from build123d import *

# Parameters (mm, degrees)
F0_R     = 45
F1_DEPTH = 8
F3_DEPTH = 25
F5_DEPTH = 25


with BuildPart() as f1:
    # F0 (on Top) → F1 (new body)
    with BuildSketch(Plane.XY):
        Circle(F0_R)
    extrude(amount=F1_DEPTH)

    # F2 (on face) → F3 (cut)
    with BuildSketch(Plane.XY.offset(8)):
        with BuildLine():
            ThreePointArc((-44.7762963998, 4.4814373498), (-31.5268148945, 32.1101221207), (-3.659898693, 44.8509213011))
            Line((-3.659898693, 44.8509213011), (-3.659898693, 46.727180481))
            Line((-3.659898693, 46.727180481), (-14.4028495997, 46.727180481))
            Line((-14.4028495997, 46.727180481), (-30.4222777486, 39.8657522048))
            Line((-30.4222777486, 39.8657522048), (-45.7375533879, 26.1307712644))
            Line((-45.7375533879, 26.1307712644), (-50.4905698847, 4.4814373498))
            Line((-50.4905698847, 4.4814373498), (-44.7762963998, 4.4814373498))
        make_face()
        with BuildLine():
            Line((-3.659898693, 39.8657522048), (-3.659898693, 44.8509213011))
            ThreePointArc((-3.659898693, 44.8509213011), (-31.5268148945, 32.1101221207), (-44.7762963998, 4.4814373498))
            Line((-44.7762963998, 4.4814373498), (-39.7817769409, 4.4814373498))
            Line((-39.7817769409, 4.4814373498), (-38.9415013432, 9.2861472328))
            Line((-38.9415013432, 9.2861472328), (-35.9457781326, 17.6231124305))
            Line((-35.9457781326, 17.6231124305), (-31.6359626456, 24.5324056053))
            Line((-31.6359626456, 24.5324056053), (-25.7671181964, 30.6386794289))
            Line((-25.7671181964, 30.6386794289), (-18.6895557962, 35.4030162759))
            Line((-18.6895557962, 35.4030162759), (-10.3150569916, 38.6816837348))
            Line((-10.3150569916, 38.6816837348), (-3.659898693, 39.8657522048))
        make_face()
        with BuildLine():
            ThreePointArc((44.7762963998, 4.4814373498), (31.5268148945, 32.1101221207), (3.659898693, 44.8509213011))
            Line((3.659898693, 44.8509213011), (3.659898693, 39.8657522048))
            Line((3.659898693, 39.8657522048), (10.3150569916, 38.6816837348))
            Line((10.3150569916, 38.6816837348), (18.6895557962, 35.4030162759))
            Line((18.6895557962, 35.4030162759), (25.7671181964, 30.6386794289))
            Line((25.7671181964, 30.6386794289), (31.6359626456, 24.5324056053))
            Line((31.6359626456, 24.5324056053), (35.9457781326, 17.6231124305))
            Line((35.9457781326, 17.6231124305), (38.9415013432, 9.2861472328))
            Line((38.9415013432, 9.2861472328), (39.7817769409, 4.4814373498))
            Line((39.7817769409, 4.4814373498), (44.7762963998, 4.4814373498))
        make_face()
        with BuildLine():
            Line((3.659898693, 46.727180481), (3.659898693, 44.8509213011))
            ThreePointArc((3.659898693, 44.8509213011), (31.5268148945, 32.1101221207), (44.7762963998, 4.4814373498))
            Line((44.7762963998, 4.4814373498), (50.4905698847, 4.4814373498))
            Line((50.4905698847, 4.4814373498), (45.7375533879, 26.1307712644))
            Line((45.7375533879, 26.1307712644), (30.4222777486, 39.8657522048))
            Line((30.4222777486, 39.8657522048), (14.4028495997, 46.727180481))
            Line((14.4028495997, 46.727180481), (3.659898693, 46.727180481))
        make_face()
        with BuildLine():
            ThreePointArc((3.659898693, -44.8509213011), (31.5268148945, -32.1101221207), (44.7762963998, -4.4814373498))
            Line((44.7762963998, -4.4814373498), (39.7817769409, -4.4814373498))
            Line((39.7817769409, -4.4814373498), (38.9415013432, -9.2861472328))
            Line((38.9415013432, -9.2861472328), (35.9457781326, -17.6231124305))
            Line((35.9457781326, -17.6231124305), (31.6359626456, -24.5324056053))
            Line((31.6359626456, -24.5324056053), (25.7671181964, -30.6386794289))
            Line((25.7671181964, -30.6386794289), (18.6895557962, -35.4030162759))
            Line((18.6895557962, -35.4030162759), (10.3150569916, -38.6816837348))
            Line((10.3150569916, -38.6816837348), (3.659898693, -39.8657522048))
            Line((3.659898693, -39.8657522048), (3.659898693, -44.8509213011))
        make_face()
        with BuildLine():
            Line((50.4905698847, -4.4814373498), (44.7762963998, -4.4814373498))
            ThreePointArc((44.7762963998, -4.4814373498), (31.5268148945, -32.1101221207), (3.659898693, -44.8509213011))
            Line((3.659898693, -44.8509213011), (3.659898693, -46.727180481))
            Line((3.659898693, -46.727180481), (14.4028495997, -46.727180481))
            Line((14.4028495997, -46.727180481), (30.4222777486, -39.8657522048))
            Line((30.4222777486, -39.8657522048), (45.7375533879, -26.1307712644))
            Line((45.7375533879, -26.1307712644), (50.4905698847, -4.4814373498))
        make_face()
        with BuildLine():
            Line((-39.7817769409, -4.4814373498), (-44.7762963998, -4.4814373498))
            ThreePointArc((-44.7762963998, -4.4814373498), (-31.5268148945, -32.1101221207), (-3.659898693, -44.8509213011))
            Line((-3.659898693, -44.8509213011), (-3.659898693, -39.8657522048))
            Line((-3.659898693, -39.8657522048), (-10.3150569916, -38.6816837348))
            Line((-10.3150569916, -38.6816837348), (-18.6895557962, -35.4030162759))
            Line((-18.6895557962, -35.4030162759), (-25.7671181964, -30.6386794289))
            Line((-25.7671181964, -30.6386794289), (-31.6359626456, -24.5324056053))
            Line((-31.6359626456, -24.5324056053), (-35.9457781326, -17.6231124305))
            Line((-35.9457781326, -17.6231124305), (-38.9415013432, -9.2861472328))
            Line((-38.9415013432, -9.2861472328), (-39.7817769409, -4.4814373498))
        make_face()
        with BuildLine():
            ThreePointArc((-3.659898693, -44.8509213011), (-31.5268148945, -32.1101221207), (-44.7762963998, -4.4814373498))
            Line((-44.7762963998, -4.4814373498), (-50.4905698847, -4.4814373498))
            Line((-50.4905698847, -4.4814373498), (-45.7375533879, -26.1307712644))
            Line((-45.7375533879, -26.1307712644), (-30.4222777486, -39.8657522048))
            Line((-30.4222777486, -39.8657522048), (-14.4028495997, -46.727180481))
            Line((-14.4028495997, -46.727180481), (-3.659898693, -46.727180481))
            Line((-3.659898693, -46.727180481), (-3.659898693, -44.8509213011))
        make_face()
    extrude(amount=-F3_DEPTH, mode=Mode.SUBTRACT)

    # F4 (on face) → F5 (cut)
    with BuildSketch(Plane.XY.offset(8)):
        with BuildLine():
            ThreePointArc((-34.7455865377, -4.4814373498), (-24.4781891298, -25.0630668813), (-3.659898693, -34.841702113))
            Line((-3.659898693, -34.841702113), (-3.659898693, -29.8095658037))
            ThreePointArc((-3.659898693, -29.8095658037), (-20.9416331367, -21.5279602707), (-29.6971680658, -4.4814373498))
            Line((-29.6971680658, -4.4814373498), (-34.7455865377, -4.4814373498))
        make_face()
        with BuildLine():
            ThreePointArc((-24.6290031955, -4.4814373498), (-17.4044615557, -17.993215307), (-3.659898693, -24.7644144022))
            Line((-3.659898693, -24.7644144022), (-3.659898693, -19.6962490835))
            ThreePointArc((-3.659898693, -19.6962490835), (-13.8659969572, -14.4592950999), (-19.5257216431, -4.4814373498))
            Line((-19.5257216431, -4.4814373498), (-24.6290031955, -4.4814373498))
        make_face()
        with BuildLine():
            ThreePointArc((-14.3499063746, -4.4814373498), (-10.3241960537, -10.9276744793), (-3.659898693, -14.5810917025))
            Line((-3.659898693, -14.5810917025), (-3.659898693, -9.342068428))
            ThreePointArc((-3.659898693, -9.342068428), (-6.769710949, -7.4054111718), (-8.9769605233, -4.4814373498))
            Line((-8.9769605233, -4.4814373498), (-14.3499063746, -4.4814373498))
        make_face()
        with BuildLine():
            Line((3.659898693, -3.4554666532), (3.659898693, 3.4554666532))
            ThreePointArc((3.659898693, 3.4554666532), (3.0196847302, 4.0269855183), (2.2916866091, 4.4814373498))
            Line((2.2916866091, 4.4814373498), (-2.2916866091, 4.4814373498))
            ThreePointArc((-2.2916866091, 4.4814373498), (-3.0196847302, 4.0269855183), (-3.659898693, 3.4554666532))
            Line((-3.659898693, 3.4554666532), (-3.659898693, -3.4554666532))
            ThreePointArc((-3.659898693, -3.4554666532), (-3.0196847302, -4.0269855183), (-2.2916866091, -4.4814373498))
            Line((-2.2916866091, -4.4814373498), (2.2916866091, -4.4814373498))
            ThreePointArc((2.2916866091, -4.4814373498), (3.0196847302, -4.0269855183), (3.659898693, -3.4554666532))
        make_face()
        with BuildLine():
            ThreePointArc((3.659898693, -14.5810917025), (10.3241960537, -10.9276744793), (14.3499063746, -4.4814373498))
            Line((14.3499063746, -4.4814373498), (8.9769605233, -4.4814373498))
            ThreePointArc((8.9769605233, -4.4814373498), (6.769710949, -7.4054111718), (3.659898693, -9.342068428))
            Line((3.659898693, -9.342068428), (3.659898693, -14.5810917025))
        make_face()
        with BuildLine():
            ThreePointArc((3.659898693, -24.7644144022), (17.4044615557, -17.993215307), (24.6290031955, -4.4814373498))
            Line((24.6290031955, -4.4814373498), (19.5257216431, -4.4814373498))
            ThreePointArc((19.5257216431, -4.4814373498), (13.8659969572, -14.4592950999), (3.659898693, -19.6962490835))
            Line((3.659898693, -19.6962490835), (3.659898693, -24.7644144022))
        make_face()
        with BuildLine():
            ThreePointArc((3.659898693, -34.841702113), (24.4781891298, -25.0630668813), (34.7455865377, -4.4814373498))
            Line((34.7455865377, -4.4814373498), (29.6971680658, -4.4814373498))
            ThreePointArc((29.6971680658, -4.4814373498), (20.9416331367, -21.5279602707), (3.659898693, -29.8095658037))
            Line((3.659898693, -29.8095658037), (3.659898693, -34.841702113))
        make_face()
        with BuildLine():
            Line((29.6971680658, 4.4814373498), (34.7455865377, 4.4814373498))
            ThreePointArc((34.7455865377, 4.4814373498), (24.4781891298, 25.0630668813), (3.659898693, 34.841702113))
            Line((3.659898693, 34.841702113), (3.659898693, 29.8095658037))
            ThreePointArc((3.659898693, 29.8095658037), (20.9416331367, 21.5279602707), (29.6971680658, 4.4814373498))
        make_face()
        with BuildLine():
            Line((19.5257216431, 4.4814373498), (24.6290031955, 4.4814373498))
            ThreePointArc((24.6290031955, 4.4814373498), (17.4044615557, 17.993215307), (3.659898693, 24.7644144022))
            Line((3.659898693, 24.7644144022), (3.659898693, 19.6962490835))
            ThreePointArc((3.659898693, 19.6962490835), (13.8659969572, 14.4592950999), (19.5257216431, 4.4814373498))
        make_face()
        with BuildLine():
            Line((8.9769605233, 4.4814373498), (14.3499063746, 4.4814373498))
            ThreePointArc((14.3499063746, 4.4814373498), (10.3241960537, 10.9276744793), (3.659898693, 14.5810917025))
            Line((3.659898693, 14.5810917025), (3.659898693, 9.342068428))
            ThreePointArc((3.659898693, 9.342068428), (6.769710949, 7.4054111718), (8.9769605233, 4.4814373498))
        make_face()
        with BuildLine():
            Line((-3.659898693, 9.342068428), (-3.659898693, 14.5810917025))
            ThreePointArc((-3.659898693, 14.5810917025), (-10.3241960537, 10.9276744793), (-14.3499063746, 4.4814373498))
            Line((-14.3499063746, 4.4814373498), (-8.9769605233, 4.4814373498))
            ThreePointArc((-8.9769605233, 4.4814373498), (-6.769710949, 7.4054111718), (-3.659898693, 9.342068428))
        make_face()
        with BuildLine():
            Line((-3.659898693, 19.6962490835), (-3.659898693, 24.7644144022))
            ThreePointArc((-3.659898693, 24.7644144022), (-17.4044615557, 17.993215307), (-24.6290031955, 4.4814373498))
            Line((-24.6290031955, 4.4814373498), (-19.5257216431, 4.4814373498))
            ThreePointArc((-19.5257216431, 4.4814373498), (-13.8659969572, 14.4592950999), (-3.659898693, 19.6962490835))
        make_face()
        with BuildLine():
            Line((-3.659898693, 29.8095658037), (-3.659898693, 34.841702113))
            ThreePointArc((-3.659898693, 34.841702113), (-24.4781891298, 25.0630668813), (-34.7455865377, 4.4814373498))
            Line((-34.7455865377, 4.4814373498), (-29.6971680658, 4.4814373498))
            ThreePointArc((-29.6971680658, 4.4814373498), (-20.9416331367, 21.5279602707), (-3.659898693, 29.8095658037))
        make_face()
    extrude(amount=-F5_DEPTH, mode=Mode.SUBTRACT)


solid = f1.part
The model under review builds one solid part; all positions refer to its coordinate system, in mm. A direction names the side the tool comes from. Coordinates: 2 decimals unless noted, no trailing zeros. Write each loop counter-clockwise with the first axis right and the second up, starting at its lowest first coordinate (ties: lowest second). Pieces come first, ordered by that corner, then holes. Notation, with made-up numbers: (86, 1) - (141, 1) arc R28 cw to (141, 21) - close; hole circle Ø10 at (-27.5, -26). An arc over 180 degrees is marked (long way). Answer as CSV lines item,"result".
(1) We need section B-B (x = -22). Give the boundary of the cut face in (y, z).
Data:
outline,"(-33.17, 0) - (-27.26, 0) - (-27.26, 8) - (-33.17, 8) - close; (-20.45, 0) - (-11.94, 0) - (-11.94, 8) - (-20.45, 8) - close; (-4.48, 0) - (4.48, 0) - (4.48, 8) - (-4.48, 8) - close; (11.94, 0) - (20.45, 0) - (20.45, 8) - (11.94, 8) - close; (27.26, 0) - (33.17, 0) - (33.17, 8) - (27.26, 8) - close"
(2) Clearance check with flat-ended pins moving along their axes: pin 1 Ø1 at (y, z) = (-7.5, 3) entering from -X; pin 2 Ø4 at (x, z) = (-43, 3.5) entering from -Y; pin 3 Ø2.5 at (y, z) = (-11.5, 5.5) entering from +X; pin 4 Ø10 at (x, y) = (-30, 25) entering from -Z. State where each tip first meets the part, or that it passes through.
Data:
pin 1,"stops at x = -39.34"
pin 2,"stops at y = -4.48"
pin 3,"stops at x = 38.6"
pin 4,"stops at z = 0"
(3) We need section D-D (y = -6.5). Give the boundary of the cut face in (x, z), plus the area to 3 significant figures.
Data:
outline,"(-39.43, 0) - (-34.43, 0) - (-34.43, 8) - (-39.43, 8) - close; (-29.32, 0) - (-24.17, 0) - (-24.17, 8) - (-29.32, 8) - close; (-18.95, 0) - (-13.56, 0) - (-13.56, 8) - (-18.95, 8) - close; (-7.64, 0) - (7.64, 0) - (7.64, 8) - (-7.64, 8) - close; (13.56, 0) - (18.95, 0) - (18.95, 8) - (13.56, 8) - close; (24.17, 0) - (29.32, 0) - (29.32, 8) - (24.17, 8) - close; (34.43, 0) - (39.43, 0) - (39.43, 8) - (34.43, 8) - close"
area,"371 mm2"
(4) Tool access review of faces 4 (the flat face through (42, 4.481, 4)), 5 (the flat face through (37.465, -13.396, 4.056)), 6 (the flat face through (-42, -4.481, 4)), 7 (the cylindrical face through (6.73, 7.44, 4.06)): name each direction out of +Z, -Z, +X, -X, +Y, -Y from which nothing blocks a thin tool from reaching the whole face with its end or side.
Data:
face 4,"+Z, -Z, +X, +Y"
face 5,"+Z, -Z, +X, -Y"
face 6,"+Z, -Z, -X, -Y"
face 7,"+Z, -Z"
(5) We need section A-A (y = -26). Give the boundary of the cut face in (x, z).
Data:
outline,"(-30.23, 0) - (-23.48, 0) - (-23.48, 8) - (-30.23, 8) - close; (-15.03, 0) - (15.03, 0) - (15.03, 8) - (-15.03, 8) - close; (23.48, 0) - (30.23, 0) - (30.23, 8) - (23.48, 8) - close"
(6) For line 1 along Y through (x, z) = (-25, 4.25); line 2 along Y through (x, z) = (21, 6); line 3 along Y through (x, z) = (-27, 1.25), list the stretches that pass through material, from the lowest coordinate up. Write a range as [from, to].
Data:
line 1,"y = [-31.16, -24.54], [-16.64, 16.64], [24.54, 31.16]"
line 2,"y = [-33.85, -28.04], [-21.47, -13.63], [-4.48, 4.48], [13.63, 21.47], [28.04, 33.85]"
line 3,"y = [-29.36, -22.32], [-13.15, 13.15], [22.32, 29.36]"
(7) Mouldability with a two-part tool opening along Y and no side actions: class faces 1 (the flat face through (-42, 4.481, 4)), 2 (the flat face through (-12, -4.481, 4)), 3 (the flat face through (42, -4.481, 4)) as pulls with the +Y half, pulls with the -Y half, needs draft (parallel to the pull), parting line crosses it, or undercut.
Data:
face 1,"pulls with the +Y half"
face 2,"undercut"
face 3,"pulls with the -Y half"
(8) We need section C-C (x = 28). Give the boundary of the cut face in (y, z).
Data:
outline,"(-28.32, 0) - (-21.06, 0) - (-21.06, 8) - (-28.32, 8) - close; (-10.86, 0) - (10.86, 0) - (10.86, 8) - (-10.86, 8) - close; (21.06, 0) - (28.32, 0) - (28.32, 8) - (21.06, 8) - close"
